Verification items for this drawing (mm, ordinates from the low corner). A direction names the side the tool comes from. Coordinates: 2 decimals unless noted, no trailing zeros. Write each loop counter-clockwise with the first axis right and the second up, starting at its lowest first coordinate (ties: lowest second). Pieces come first, ordered by that corner, then holes.
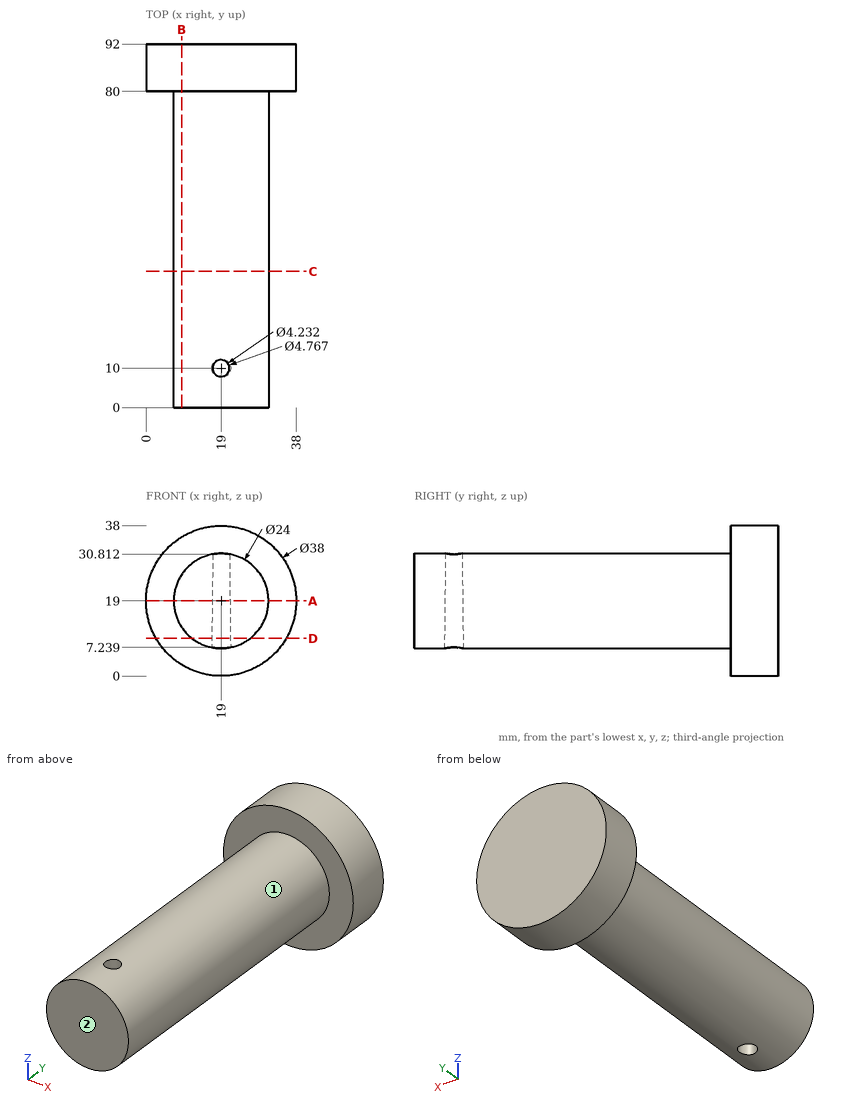
1. Gauge pin test, flat ends, axial feed: pin 1 Ø4 at (y, z) = (23, 27) entering from +X; pin 2 Ø12 at (x, y) = (34, 58) entering from +Z; pin 3 Ø12 at (y, z) = (64, 29.5) entering from -X (1 decimal). Record the tip position at first contact, or that the pin passes through.
Computed values:
pin 1: stops at x = 29.39
pin 2: stops at z = 26.94
pin 3: stops at x = 7.9
2. Access from +Z, -Z, +X, -X, +Y, -Y to the whole of each face (thin tool, end or side, straight path). Record for the marked faces 1 and 2.
Computed values:
face 1: -Y
face 2: +Z, -Z, +X, -X, -Y
3. Sectioned sample at D-D, the plane z = 9.5. Record the boundary of the cut face in (x, y) (1 decimal).
Computed values:
outline: (2.5, 80) - (11.7, 80) - (11.7, 0) - (26.3, 0) - (26.3, 80) - (35.5, 80) - (35.5, 92) - (2.5, 92) - close; hole circle Ø4.7 at (19, 10)
4. Sectioned sample at C-C, the plane y = 34.5. Record the boundary of the cut face in (x, z).
Computed values:
outline: circle Ø24 at (19, 19)
5. Sectioned sample at B-B, the plane x = 9. Record the boundary of the cut face in (y, z) (1 decimal), and give its area (3 significant figures).
Computed values:
outline: (0, 12.4) - (80, 12.4) - (80, 2.8) - (92, 2.8) - (92, 35.2) - (80, 35.2) - (80, 25.6) - (0, 25.6) - close
area: 1,450 mm2
6. Sectioned sample at A-A, the plane z = 19. Record the boundary of the cut face in (x, y).
Computed values:
outline: (0, 80) - (7, 80) - (7, 0) - (31, 0) - (31, 80) - (38, 80) - (38, 92) - (0, 92) - close; hole circle Ø4.5 at (19, 10)
7. Thickness scan on line 1 along Y through (x, z) = (26, 7); line 2 along Y through (x, z) = (21, 19.5) (1 decimal); line 3 along Z through (x, y) = (21, 15). Record the ranges inside material, lowest first.
Computed values:
line 1: y = 80 to 92
line 2: y = 0 to 9, 11 to 92
line 3: z = 7.17 to 30.83
